Here's the drawing with two shaded views (mm, measured from the low corner). I have some questions. Give positions to 0.01 mm unless a question says otherwise; leave off trailing zeros. Write each loop counter-clockwise with the first axis right and the second up, starting at its lowest first coordinate (ties: lowest second). Pieces come first, ordered by that corner, then holes. Notation, with made-up numbers: M -39,-6 L -22,-6 A22 ccw -22,17 Z; hole C 69,58.5 d11. An arc over 180 degrees is marked long. Use one line per item in the form item = value.
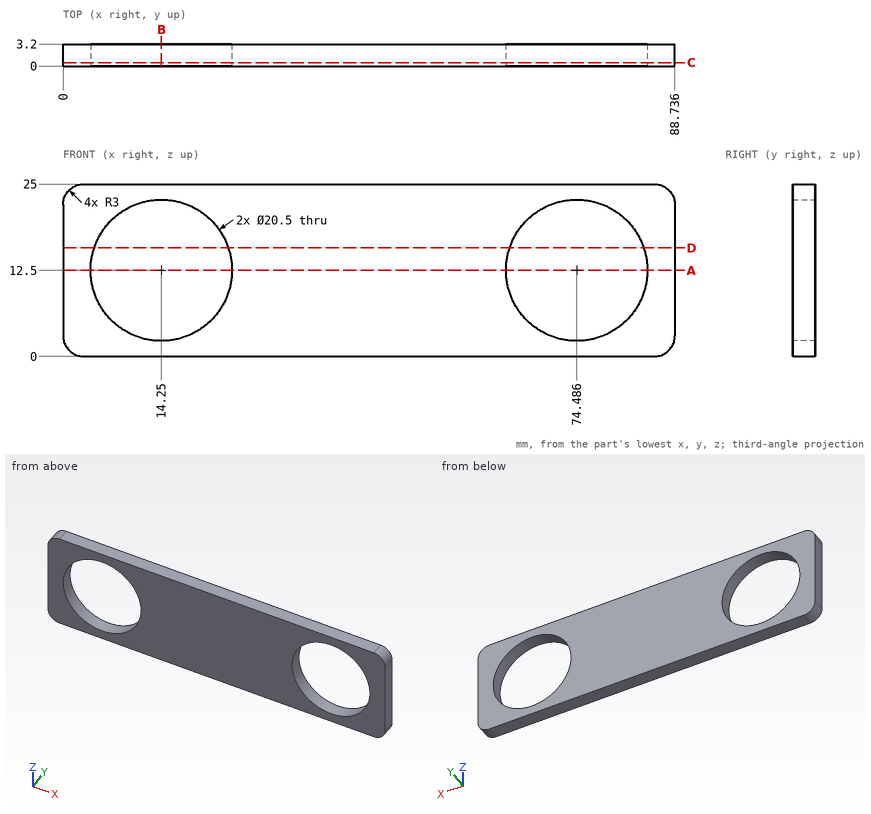
1) I want a section at A-A, the plane z = 12.5. Please give me the cut outline in (x, y).
Checked values:
outline = M 0,0 L 4,0 L 4,3.2 L 0,3.2 Z; M 24.5,0 L 64.24,0 L 64.24,3.2 L 24.5,3.2 Z; M 84.74,0 L 88.74,0 L 88.74,3.2 L 84.74,3.2 Z
2) If I drill on L1, parallel to X at y = 2.35, z = 12.5; L2, parallel to X at y = 0.65, z = 14.75; L3, parallel to Z at x = 14.5, y = 1.9, over which ranges is the centre line in solid material (lowest first)?
Checked values:
L1 = 0 to 4, 24.5 to 64.24, 84.74 to 88.74
L2 = 0 to 4.25, 24.25 to 64.49, 84.49 to 88.74
L3 = 0 to 2.25, 22.75 to 25
3) I want a section at D-D, the plane z = 15.75. Please give me the cut outline in (x, y), plus the area to 3 significant figures.
Checked values:
outline = M 0,0 L 4.53,0 L 4.53,3.2 L 0,3.2 Z; M 23.97,0 L 64.76,0 L 64.76,3.2 L 23.97,3.2 Z; M 84.21,0 L 88.74,0 L 88.74,3.2 L 84.21,3.2 Z
area = 160 mm2
4) For pin 1 Ø5 at (x, z) = (24.5, 21) entering from -Y, with a flat end and sliding along its axis, tell me the tip position at first contact or that it passes through.
Checked values:
pin_1 = 0
5) I want a section at B-B, the plane x = 14.25. Please give me the cut outline in (y, z).
Checked values:
outline = M 0,0 L 3.2,0 L 3.2,2.25 L 0,2.25 Z; M 0,22.75 L 3.2,22.75 L 3.2,25 L 0,25 Z
6) I want a section at C-C, the plane y = 0.5. Please give me the cut outline in (x, z), plus the area to 3 significant figures.
Checked values:
outline = M 0,3 A3 ccw 3,0 L 85.74,0 A3 ccw 88.74,3 L 88.74,22 A3 ccw 85.74,25 L 3,25 A3 ccw 0,22 Z; hole C 14.25,12.5 d20.5; hole C 74.49,12.5 d20.5
area = 1,550 mm2
